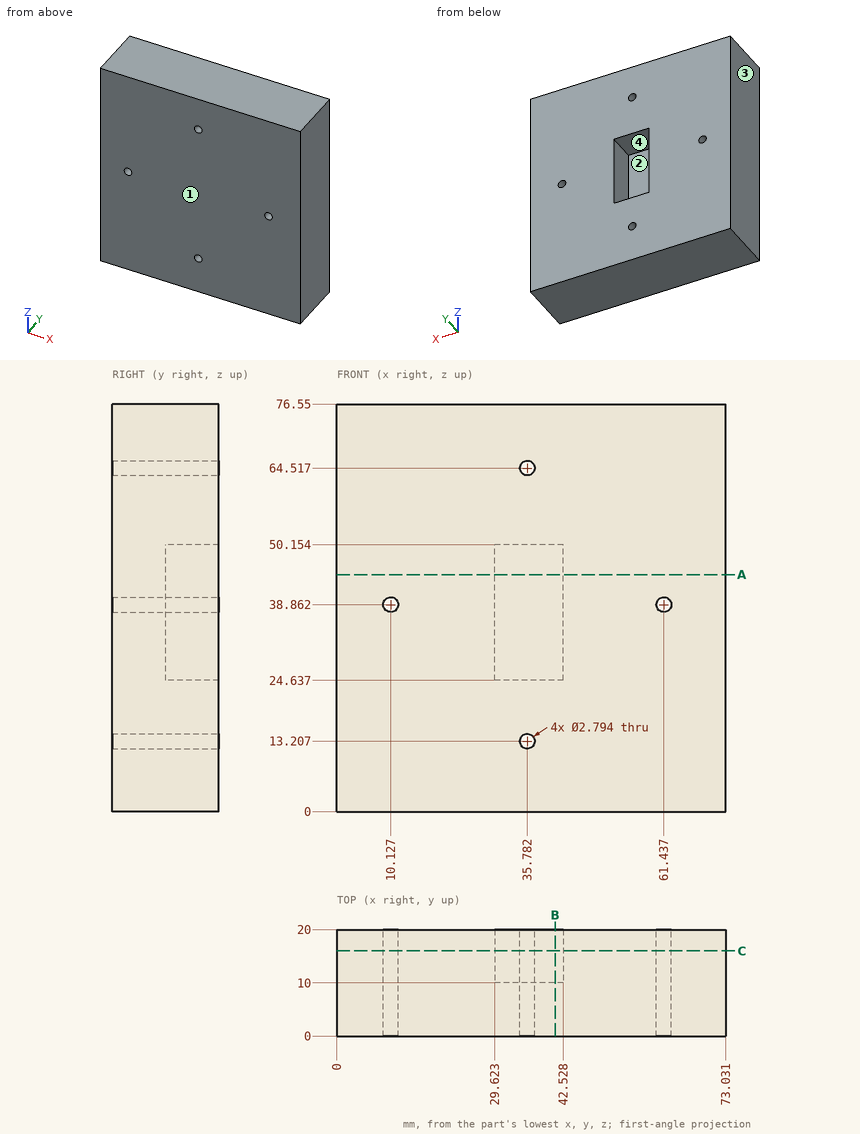
The figure shows three views and two pictorial views of one solid part (mm, origin at its lowest corner). Answer the questions. Coordinates: 2 decimals unless noted, no trailing zeros. Order: outer loops, then holes, each group sorted by start corner. A loop starts at its lowest first (then second) coordinate and runs counter-clockwise, first axis right, second up.
Q1. Consider line 1 (X direction, y = 15.25, z = 49); line 2 (X direction, y = 15.25, z = 13); line 3 (X direction, y = 18.5, z = 38) (1 decimal). Determine where each line is inside the solid, lowest interval first.
Q2. A cutting plane is placed at C-C, the plane y = 16. State how many separate pieces and enclosed holes the cut face has, and give its area (3 significant figures).
Q3. For a pull along X with two mould halves and no side action, classify the marked faces 1, 2, 3 and 4 as pulls with the +X half, pulls with the -X half, needs draft (parallel to the pull), parting line crosses it, or undercut.
Q4. Given P1, Ø11, axis at x = 39, y = 14.5, coming from the -Z side; P2, Ø1.7, axis at x = 35.78, z = 64.52, coming from the +Y side, each flat-ended and moving along its own axis, determine where each tip first touches the part or whether it passes through.
Q5. A cutting plane is placed at A-A, the plane z = 44.5. Write down the section's boundary in (x, y).
Q6. A cutting plane is placed at B-B, the plane x = 41. Write down the section's boundary in (y, z).
Answers follow:
1. line 1: x = 0 to 29.62, 42.53 to 73.03
1. line 2: x = 0 to 34.4, 37.16 to 73.03
1. line 3: x = 0 to 9, 11.2 to 29.6, 42.5 to 60.3, 62.5 to 73
2. separate pieces: 1
2. enclosed holes: 5
2. area: 5,240 mm2
3. face 1: needs draft
3. face 2: undercut
3. face 3: pulls with the -X half
3. face 4: undercut
4. P1: stops at z = 0
4. P2: passes through
5. outline: (0, 0) - (73.03, 0) - (73.03, 20) - (42.53, 20) - (42.53, 10) - (29.62, 10) - (29.62, 20) - (0, 20) - close
6. outline: (0, 0) - (20, 0) - (20, 24.64) - (10, 24.64) - (10, 50.15) - (20, 50.15) - (20, 76.55) - (0, 76.55) - close
